Could you check a few things on this drawing? It's one solid part, dimensions in mm from its lowest x, y, z. Coordinates: 2 decimals unless noted, no trailing zeros. Order: outer loops, then holes, each group sorted by start corner. A loop starts at its lowest first (then second) coordinate and runs counter-clockwise, first axis right, second up. Notation, with made-up numbers: (42, -3) - (59, -3) arc R25 cw to (59, 9) - close; hole circle Ø2 at (62.25, 21). An arc over 180 degrees is marked (long way). Answer in a Markdown table with one row per item. Add a question column.
Item 1: Will this pin go through, and if not, where does the flat tip stop? pin 1 Ø2.5 at (x, y) = (2.5, 40.25) entering from -Z.
Item 2: I want a section at B-B (x = 2.5). Please give me the cut outline in (y, z), plus the area to 3 significant figures.
Item 3: If I drill on line 1 along X through (y, z) = (7.5, 0.9); line 2 along Y through (x, z) = (97.5, 0.75); line 3 along Y through (x, z) = (96.5, 1.1), over which ranges is the centre line in solid material (lowest first)? Write a range as from..to.
Item 4: I want a section at A-A (y = 40.25). Please give me the cut outline in (x, z).
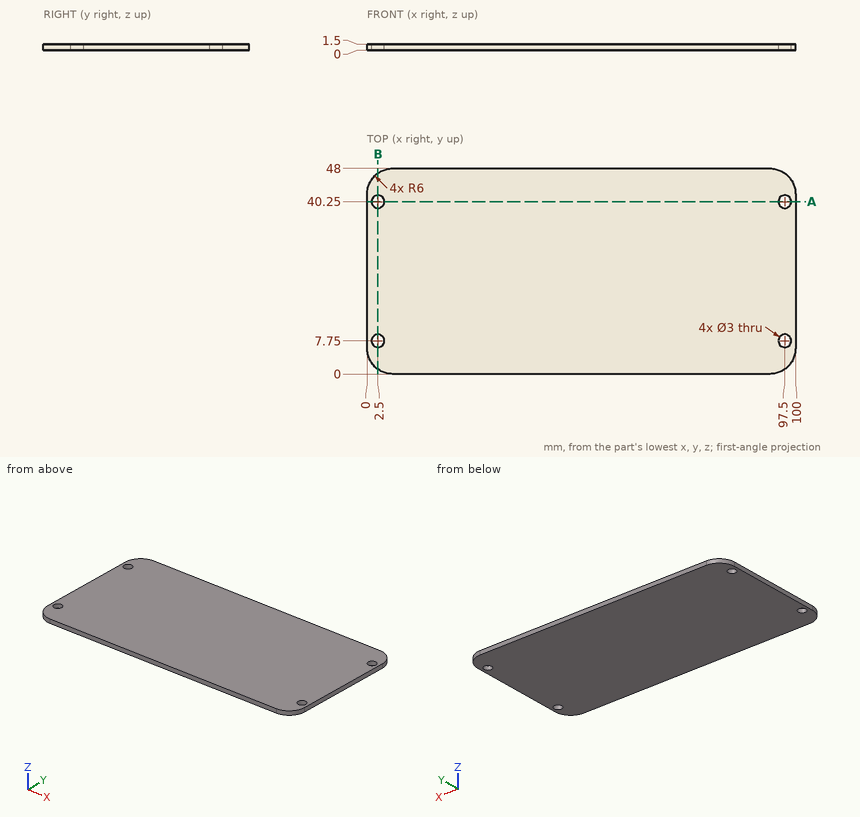
Values follow:
| question | item | result |
|---|---|---|
| 1 | pin 1 | passes through |
| 2 | outline | (1.13, 0) - (6.25, 0) - (6.25, 1.5) - (1.13, 1.5) - close; (9.25, 0) - (38.75, 0) - (38.75, 1.5) - (9.25, 1.5) - close; (41.75, 0) - (46.87, 0) - (46.87, 1.5) - (41.75, 1.5) - close |
| 2 | area | 59.6 mm^2 |
| 3 | line 1 | x = 0..1.02, 3.98..96.02, 98.98..100 |
| 3 | line 2 | y = 1.13..6.25, 9.25..38.75, 41.75..46.87 |
| 3 | line 3 | y = 0.55..6.63, 8.87..39.13, 41.37..47.45 |
| 4 | outline | (0, 0) - (1, 0) - (1, 1.5) - (0, 1.5) - close; (4, 0) - (96, 0) - (96, 1.5) - (4, 1.5) - close; (99, 0) - (100, 0) - (100, 1.5) - (99, 1.5) - close |
